The listing builds one solid part. Answer for the finished solid, in the listing's coordinates (mm). Coordinates: 2 decimals unless noted, no trailing zeros.
(1) The part is cut by section A-A on z = 859.5. Give the number of separate pieces and of enclosed holes in the cut face, plus the area to 3 significant figures.
(2) Straight lines are drawn through the part: line 1 (Y direction, x = 8, z = 732); line 2 (Y direction, x = 0, z = 380); line 3 (X direction, y = 5, z = 179). For each, find the intervals that lie inside material, in ascending order.
(3) Given P1, Ø0.8, axis at y = 3.5, z = 711.5, coming from the +X side; P2, Ø1.7, axis at x = 1, z = 637, coming from the -Y side; P3, Ø4.5, axis at y = 0.5, z = 672, coming from the +X side, each flat-ended and moving along its own axis, determine where each tip first touches the part or whether it passes through.
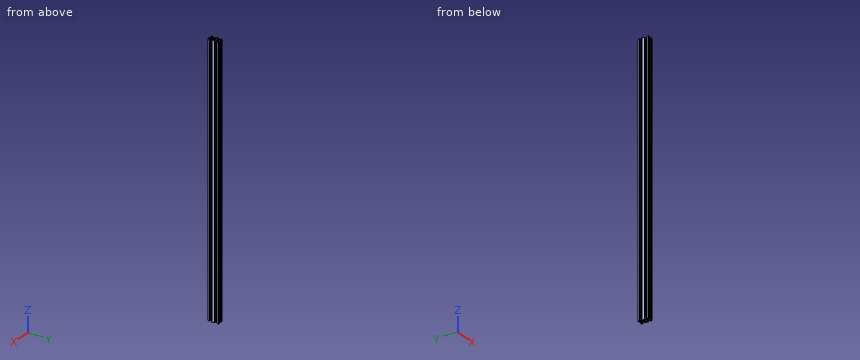
Autodesk Inventor part; units mm, degrees
ref_plane "Work Plane1" through (0, -10, 0) normal (0, 1, 0) x (-1, 0, 0)
ref_plane "YZ Plane" through (0, 0, 0) normal (1, 0, 0) x (0, 1, 0)
ref_plane "XY Plane" through (0, 0, 0) normal (0, 0, 1) x (1, 0, 0)
sketch "Sketch1" plane through (0, 0, 0) normal (0, 0, 1) x (1, 0, 0)
  line L0 (-3.9007, 3.9007) -> (3.9007, 3.9007)
  line L1 (3.9007, 3.9007) -> (3.9007, -3.9007)
  line L2 (3.9007, -3.9007) -> (-3.9007, -3.9007)
  line L3 (-3.9007, -3.9007) -> (-3.9007, 3.9007)
  line L4 (0, 3.9007) -> (0, -3.9007) construction
  line L5 (-3.9007, 0) -> (3.9007, 0) construction
  circle A0 centre (0, 0) radius 2.1
  line L6 (0, 0) -> (-16.1173, 16.1173) construction
  line L7 (0, 0) -> (22.7933, 0) construction
  line L8 (-2.84, 3.9007) -> (-5.4993, 6.56)
  line L9 (-5.4993, 6.56) -> (-5.4993, 8.2)
  line L10 (-5.4993, 8.2) -> (-2.84, 8.2)
  line L11 (-2.84, 8.2) -> (-4.64, 10)
  line L12 (-4.64, 10) -> (-10, 10)
  line L13 (-10, 10) -> (-10, 4.64)
  line L14 (-10, 4.64) -> (-8.2, 2.84)
  line L15 (-8.2, 2.84) -> (-8.2, 5.4993)
  line L16 (-8.2, 5.4993) -> (-6.56, 5.4993)
  line L17 (-6.56, 5.4993) -> (-3.9007, 2.84)
  line L18 (-3.9007, 2.84) -> (-11.3102, 2.84) construction
  line L19 (-2.84, 3.9007) -> (-3.9007, 3.9007)
  line L20 (-3.9007, 2.84) -> (-3.9007, 3.9007)
  line L21 (-3.9007, -2.84) -> (-6.56, -5.4993)
  line L22 (-6.56, -5.4993) -> (-8.2, -5.4993)
  line L23 (-8.2, -5.4993) -> (-8.2, -2.84)
  line L24 (-8.2, -2.84) -> (-10, -4.64)
  line L25 (-10, -4.64) -> (-10, -10)
  line L26 (-10, -10) -> (-4.64, -10)
  line L27 (-4.64, -10) -> (-2.84, -8.2)
  line L28 (-2.84, -8.2) -> (-5.4993, -8.2)
  line L29 (-5.4993, -8.2) -> (-5.4993, -6.56)
  line L30 (-5.4993, -6.56) -> (-2.84, -3.9007)
  line L31 (-3.9007, -2.84) -> (-3.9007, -3.9007)
  line L32 (-2.84, -3.9007) -> (-3.9007, -3.9007)
  line L33 (2.84, -3.9007) -> (5.4993, -6.56)
  line L34 (5.4993, -6.56) -> (5.4993, -8.2)
  line L35 (5.4993, -8.2) -> (2.84, -8.2)
  line L36 (2.84, -8.2) -> (4.64, -10)
  line L37 (4.64, -10) -> (10, -10)
  line L38 (10, -10) -> (10, -4.64)
  line L39 (10, -4.64) -> (8.2, -2.84)
  line L40 (8.2, -2.84) -> (8.2, -5.4993)
  line L41 (8.2, -5.4993) -> (6.56, -5.4993)
  line L42 (6.56, -5.4993) -> (3.9007, -2.84)
  line L43 (2.84, -3.9007) -> (3.9007, -3.9007)
  line L44 (3.9007, -2.84) -> (3.9007, -3.9007)
  line L45 (3.9007, 2.84) -> (6.56, 5.4993)
  line L46 (6.56, 5.4993) -> (8.2, 5.4993)
  line L47 (8.2, 5.4993) -> (8.2, 2.84)
  line L48 (8.2, 2.84) -> (10, 4.64)
  line L49 (10, 4.64) -> (10, 10)
  line L50 (10, 10) -> (4.64, 10)
  line L51 (4.64, 10) -> (2.84, 8.2)
  line L52 (2.84, 8.2) -> (5.4993, 8.2)
  line L53 (5.4993, 8.2) -> (5.4993, 6.56)
  line L54 (5.4993, 6.56) -> (2.84, 3.9007)
  line L55 (3.9007, 2.84) -> (3.9007, 3.9007)
  line L56 (2.84, 3.9007) -> (3.9007, 3.9007)
  dimension "d7" = 4.2
  dimension "d8" = 135
  dimension "d9" = 1.5
  dimension "d10" = 1.64
  dimension "d11" = 1.8
  dimension "d12" = 2.84
  dimension "d13" = 10
  dimension "d16" = 360
extrude "Extrusion1" add sketch "Sketch1" along normal blind 1000
pattern_linear "Rectangular Pattern1" count 2 spacing 20 along (0, -1, 0) of "Extrusion1"
sketch "Sketch2" plane through (0, 0, 1000) normal (0, 0, 1) x (1, 0, 0)
  line L0 (8.2, -2.84) -> (8.2, -5.4993)
  line L1 (8.2, -5.4993) -> (6.56, -5.4993)
  line L2 (-6.56, -5.4993) -> (-8.2, -5.4993)
  line L3 (-8.2, -5.4993) -> (-8.2, -2.84)
  line L4 (-8.2, -14.5007) -> (-6.56, -14.5007)
  line L5 (6.56, -14.5007) -> (8.2, -14.5007)
  line L6 (5.4993, -11.8) -> (5.4993, -13.44)
  line L7 (5.4993, -13.44) -> (2.84, -16.0993)
  line L8 (-2.84, -16.0993) -> (-5.4993, -13.44)
  line L9 (-5.4993, -8.2) -> (-5.4993, -6.56)
  line L10 (-5.4993, -6.56) -> (-2.84, -3.9007)
  line L11 (2.84, -3.9007) -> (5.4993, -6.56)
  line L12 (2.84, -8.2) -> (4.64, -10)
  line L13 (-8.2, -6.9993) -> (-5.9387, -6.9993)
  line L14 (-5.9387, -6.9993) -> (-4.1231, -5.1837)
  line L15 (-4.1231, -5.1837) -> (4.1231, -5.1837)
  line L16 (4.1231, -5.1837) -> (5.9387, -6.9993)
  line L17 (5.9387, -6.9993) -> (8.2, -6.9993)
  line L18 (8.2, -6.9993) -> (8.2, -13.0007)
  line L19 (8.2, -13.0007) -> (5.9387, -13.0007)
  line L20 (5.9387, -13.0007) -> (4.2461, -14.6932)
  line L21 (4.2461, -14.6932) -> (-4.2461, -14.6932)
  line L22 (-4.2461, -14.6932) -> (-5.9387, -13.0007)
  line L23 (-5.9387, -13.0007) -> (-8.2, -13.0007)
  line L24 (-8.2, -13.0007) -> (-8.2, -6.9993)
  dimension "d23" = 1.5
  dimension "d24" = 1.5
  dimension "d25" = 1.5
  dimension "d26" = 1.5
extrude "Extrusion2" cut sketch "Sketch2" against normal up to next
ref_plane "Work Plane1" through (0, -10, 0) normal (0, 1, 0) x (-1, 0, 0)
equation "\"d24\" = d23"
equation "\"d25\" = d23"
equation "\"d26\" = d23"
properties part number "20x40x1000mm" material "Aluminum 6061"
Model answer:
1. separate pieces: 1
1. enclosed holes: 3
1. area: 297 mm2
2. line 1: y = -30 to -25.5, -14.5 to -13, -7 to -5.5, 5.5 to 10
2. line 2: y = -23.9 to -22.1, -17.9 to -16.1, -3.9 to -2.1, 2.1 to 3.9
2. line 3: x = -10 to -8.2, -6.06 to -3.94, 3.94 to 6.06, 8.2 to 10
3. P1: stops at x = 9.26
3. P2: stops at y = -23.9
3. P3: stops at x = 3.9
